```python
from build123d import *

# Parameters (mm, degrees)
BOSS_EXTRUDE1_DEPTH = 5
SKETCH2_W           = 2.5
SKETCH2_H           = 9.100970889
BOSS_EXTRUDE2_DEPTH = 5
CUT_EXTRUDE1_REACH  = 4.5
SKETCH3_R           = 2.7


with BuildPart() as part:
    # Sketch1 → Boss-Extrude1 (new body)
    with BuildSketch(Plane(origin=(0, 0, 0), x_dir=(1, 0, 0), z_dir=(0, 1, 0))):
        with BuildLine():
            Line((-2.5, -30.899029111), (-2.5, -24.874685928))
            ThreePointArc((-2.5, -24.874685928), (-25, 0), (-2.5, 24.874685928))
            Line((-2.5, 24.874685928), (-2.5, 30.899029111))
            ThreePointArc((-2.5, 30.899029111), (-31, 0), (-2.5, -30.899029111))
        make_face()
        with BuildLine():
            Line((0, -31), (0, -25))
            ThreePointArc((0, -25), (-1.251569376, -24.968651828), (-2.5, -24.874685928))
            Line((-2.5, -24.874685928), (-2.5, -30.899029111))
            ThreePointArc((-2.5, -30.899029111), (-1.251019097, -30.974746992), (0, -31))
        make_face()
        with BuildLine():
            Line((0, -40), (0, -31))
            ThreePointArc((0, -31), (-1.251019097, -30.974746992), (-2.5, -30.899029111))
            Line((-2.5, -30.899029111), (-2.5, -40))
            Line((-2.5, -40), (0, -40))
        make_face()
        with BuildLine():
            Line((-2.5, 30.899029111), (-2.5, 24.874685928))
            ThreePointArc((-2.5, 24.874685928), (-1.251569376, 24.968651828), (0, 25))
            Line((0, 25), (0, 31))
            ThreePointArc((0, 31), (-1.251019097, 30.974746992), (-2.5, 30.899029111))
        make_face()
        with BuildLine():
            Line((-2.5, 40), (-2.5, 30.899029111))
            ThreePointArc((-2.5, 30.899029111), (-1.251019097, 30.974746992), (0, 31))
            Line((0, 31), (0, 40))
            Line((0, 40), (-2.5, 40))
        make_face()
    extrude(amount=BOSS_EXTRUDE1_DEPTH)

    # Sketch2 → Boss-Extrude2 (add)
    with BuildSketch(Plane(origin=(0, 5, 0), x_dir=(1, 0, 0), z_dir=(0, 1, 0))):
        with Locations((-1.25, 35.449514556)):
            Rectangle(SKETCH2_W, SKETCH2_H)
        with Locations((-1.25, -35.449514556)):
            Rectangle(SKETCH2_W, SKETCH2_H)
    extrude(amount=BOSS_EXTRUDE2_DEPTH)

    # Sketch3 → Cut-Extrude1 (cut, up to next)
    with BuildSketch(Plane.ZY.offset(2.5), mode=Mode.PRIVATE) as cut_extrude1_sk1:
        with Locations((-35.449514555, 5)):
            Circle(SKETCH3_R)
    cut_extrude1_tool1 = extrude(cut_extrude1_sk1.sketch, amount=-CUT_EXTRUDE1_REACH, mode=Mode.PRIVATE) & part.part
    add(cut_extrude1_tool1.solids().sort_by_distance((-2.5, 5, -35.449515))[0], mode=Mode.SUBTRACT)
    # Sketch3 → Cut-Extrude1 (cut, up to next)
    with BuildSketch(Plane.ZY.offset(2.5), mode=Mode.PRIVATE) as cut_extrude1_sk2:
        with Locations((35.449514555, 5)):
            Circle(SKETCH3_R)
    cut_extrude1_tool2 = extrude(cut_extrude1_sk2.sketch, amount=-CUT_EXTRUDE1_REACH, mode=Mode.PRIVATE) & part.part
    add(cut_extrude1_tool2.solids().sort_by_distance((-2.5, 5, 35.449515))[0], mode=Mode.SUBTRACT)


solid = part.part
```
Here's how the part is built. I have some questions about the finished solid (model axes, mm). A direction names the side the tool comes from. Give positions to 0.01 mm unless a question says otherwise; leave off trailing zeros. Loops run counter-clockwise (first coordinate to the right, second up) from the corner with the lowest first, then second, coordinate; pieces in that order, holes last. Notation, with made-up numbers: M 77,82 L 117,82 A22 cw 117,101 Z; hole C 51.5,-6 d5. An arc over 180 degrees is marked long. Put each result on its own line as item: value. Start each with the question number.
(1) If we mould it in two halves opening along Z, with no side actions, what happens to faces 4 (the cylindrical face through (-30.993, 2.465, -0.647)), 5 (the flat face through (-1, 10, 35)), 6 (the cylindrical face through (-1.268, 5.811, -32.874))? For each: +Z half, -Z half, draft (parallel to the pull), parting line (faces both ways), or undercut.
(2) I want a section at A-A on x = -21. Please give me the cut outline in (y, z), then the cut area to 3 significant figures.
(3) I want a section at D-D on x = -17. Please give me the cut outline in (y, z).
(4) For faces 1 (the flat face through (-1, 7, -30.899)), 2 (the flat face through (-2.5, 3, -33)), 3 (the flat face through (-2.5, 3, 33)), which set-ups out of +Z, -Z, +X, -X, +Y, -Y let a thin tool reach every point of the face, with its end or its side?
(5) I want a section at B-B on y = 1.5. Please give me the cut outline in (x, z), then the cut area to 3 significant figures.
(6) I need wall thicknesses on line 1 along X through (y, z) = (8.75, -32); line 2 along Z through (x, y) = (-10, 2); line 3 along Y through (x, z) = (-27.5, -12.5). Which ranges of each line are inside material? Lowest first, please. Write a range as [from, to].
(7) Will these pins go through, and if not, where does the flat tip stop? pin 1 Ø6 at (x, y) = (-16.5, 1.5) entering from -Z; pin 2 Ø5 at (y, z) = (4.5, 10) entering from +X; pin 3 Ø5 at (x, y) = (-5.5, 7) entering from -Z.
(8) I want a section at C-C on z = 32. Please give me the cut outline in (x, y), then the cut area to 3 significant figures.
Answer block:
1. face 4: parting line
1. face 5: draft
1. face 6: undercut
2. outline: M 0,-22.8 L 5,-22.8 L 5,-13.56 L 0,-13.56 Z; M 0,13.56 L 5,13.56 L 5,22.8 L 0,22.8 Z
2. area: 92.4 mm^2
3. outline: M 0,-25.92 L 5,-25.92 L 5,-18.33 L 0,-18.33 Z; M 0,18.33 L 5,18.33 L 5,25.92 L 0,25.92 Z
4. face 1: +X, -X, +Y
4. face 2: -Z, -X, +Y, -Y
4. face 3: +Z, -X, +Y, -Y
5. outline: M -2.5,-40 L 0,-40 L 0,-25 A25 cw 0,25 L 0,40 L -2.5,40 L -2.5,30.9 A31 ccw -2.5,-30.9 Z
5. area: 573 mm^2
6. line 1: [-2.5, 0]
6. line 2: [-29.34, -22.91], [22.91, 29.34]
6. line 3: [0, 5]
7. pin 1: z = -27.91
7. pin 2: x = -21.65
7. pin 3: z = -30.74
8. outline: M -2.5,0 L 0,0 L 0,10 L -2.5,10 Z
8. area: 25.0 mm^2
